from build123d import *

# Parameters (mm, degrees)
CROQUIS1_R              = 1.6
SALIENTE_EXTRUIR1_DEPTH = 2
CROQUIS2_R              = 4
SALIENTE_EXTRUIR2_DEPTH = 11
REDONDEO1_R             = 4
REDONDEO2_R             = 4


with BuildPart() as part:
    # Croquis1 → Saliente-Extruir1 (new body)
    with BuildSketch(Plane.XY):
        Polygon((-6.5, 28), (-6.5, -8), (-2.5, -8), (-2.5, -19.4), (-11, -19.4), (-11, -28), (11, -28), (11, -19.4), (2.5, -19.4), (2.5, -8), (6.5, -8), (6.5, 28), align=None)
        with Locations((-8, -22.4)):
            Circle(CROQUIS1_R, mode=Mode.SUBTRACT)
        with Locations((8, -22.4)):
            Circle(CROQUIS1_R, mode=Mode.SUBTRACT)
    extrude(amount=SALIENTE_EXTRUIR1_DEPTH)

    # Croquis2 → Saliente-Extruir2 (add)
    with BuildSketch(Plane.XY.offset(2)):
        with Locations((0, 21.5)):
            Circle(CROQUIS2_R)
        with Locations((0, 10.3)):
            Circle(CROQUIS2_R)
        with Locations((0, -0.9)):
            Circle(CROQUIS2_R)
    extrude(amount=SALIENTE_EXTRUIR2_DEPTH)

    # Redondeo1
    redondeo1_edges = [part.edges().sort_by_distance(p)[0] for p in [
        (-4, 21.5, 13),
    ]]
    fillet(redondeo1_edges, radius=REDONDEO1_R)

    # Redondeo2
    redondeo2_edges = [part.edges().sort_by_distance(p)[0] for p in [
        (-4, 10.3, 13),
        (-4, -0.9, 13),
    ]]
    fillet(redondeo2_edges, radius=REDONDEO2_R)


solid = part.part
Geometry: final body of the model. Coordinates: model frame, mm. A direction names the side the tool comes from. Coordinates: 2 decimals unless noted, no trailing zeros. Loops run counter-clockwise (first coordinate to the right, second up) from the corner with the lowest first, then second, coordinate; pieces in that order, holes last. Notation, with made-up numbers: M -2,67.5 L 2,67.5 A17 cw 2,98.5 Z; hole C 29,6.25 d5. An arc over 180 degrees is marked long. One line per item, written item: value. Start each with the question number.
1) Pin query (flat end, axial travel): P1, Ø3, axis at x = 4.5, z = 6.5, coming from the -Y side; P2, Ø1, axis at y = 15.5, z = 1.5, coming from the -X side; P3, Ø1.6, axis at y = -14.5, z = 1.5, coming from the +X side; P4, Ø1.9, axis at x = -8, y = -22.4, coming from the +Z side. Return the tip coordinate at first contact, or that it passes through.
2) Material intervals for L1, parallel to Y at x = -8, z = 0.9; L2, parallel to Y at x = -3.5, z = 5.75; L3, parallel to Z at x = -2, y = -7.5, sorted ascending. Write a range as from..to.
3) Reachability of faces 1 (the flat face through (-2.5, -14, 1)), 2 (the flat face through (2.5, -14, 1)), 3 (the cylindrical face through (-0.521, 25.466, 5.451)), 4 (the flat face through (6.5, 10, 1)) from +Z, -Z, +X, -X, +Y, -Y: full face, straight path, thin tool, end or side. Return the list, or none.
4) Cut plane B-B (z = 5.75). Return loops of the section in (x, y), then the cut area to 3 significant figures.
5) Cut plane D-D (x = 0). Return loops of the section in (y, z), then the cut area to 3 significant figures.
6) Draft query along Y for faces 5 (the flat face through (7, -19.4, 1)), 6 (the flat face through (-6.5, 10, 1)), 7 (the flat face through (0, 28, 1)), 8 (the flat face through (0, -28, 1)). Return one class per face: released by +Y, released by -Y, zero draft, split by the parting line, or undercut.
7) Cut plane C-C (y = 21.5). Return loops of the section in (x, z).
8) Cut plane A-A (x = 8). Return loops of the section in (y, z), then the cut area to 3 significant figures.
Evaluation:
1. P1: y = -3.55
1. P2: x = -6.5
1. P3: x = 2.5
1. P4: through
2. L1: -28..-24, -20.8..-19.4
2. L2: -2.84..1.04, 8.36..12.24, 19.56..23.44
2. L3: 0..2
3. face 1: +Z, -Z, -X
3. face 2: +Z, -Z, +X
3. face 3: +Z
3. face 4: +Z, -Z, +X, +Y
4. outline: C 0,-0.9 d8; C 0,10.3 d8; C 0,21.5 d8
4. area: 151 mm^2
5. outline: M -28,0 L 28,0 L 28,2 L 25.5,2 L 25.5,9 A4 ccw 17.5,9 L 17.5,2 L 14.3,2 L 14.3,9 A4 ccw 6.3,9 L 6.3,2 L 3.1,2 L 3.1,9 A4 ccw -4.9,9 L -4.9,2 L -28,2 Z
5. area: 355 mm^2
6. face 5: undercut
6. face 6: zero draft
6. face 7: released by +Y
6. face 8: released by -Y
7. outline: M -6.5,0 L 6.5,0 L 6.5,2 L 4,2 L 4,9 A4 ccw -4,9 L -4,2 L -6.5,2 Z
8. outline: M -28,0 L -24,0 L -24,2 L -28,2 Z; M -20.8,0 L -19.4,0 L -19.4,2 L -20.8,2 Z
8. area: 10.8 mm^2
